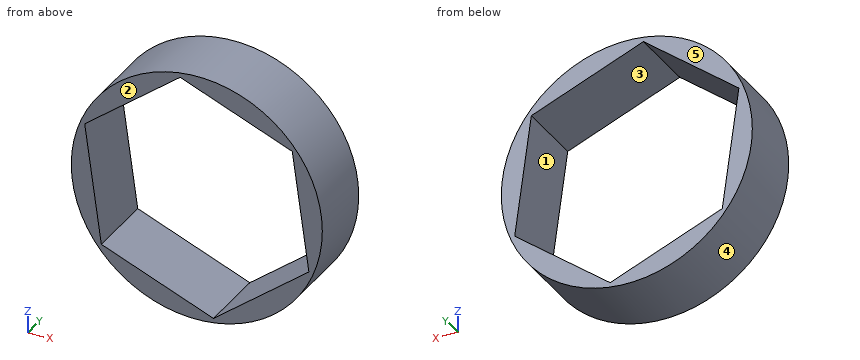
from build123d import *

# Parameters (mm, degrees)
F0_R     = 18
F1_DEPTH = 10


with BuildPart() as f1:
    # F0 (on Front) → F1 (new body)
    with BuildSketch(Plane.XZ):
        Circle(F0_R)
        Polygon((-16.075068, 6.526333), (-2.385564, 17.184584), (13.689504, 10.658251), (16.075068, -6.526333), (2.385564, -17.184584), (-13.689504, -10.658251), align=None, mode=Mode.SUBTRACT)
    extrude(amount=-F1_DEPTH)


solid = f1.part
Check sheet for the modelled part. Datum: model origin and axes. Units: mm. Face numbers are marked on the shaded views. A direction names the side the tool comes from. Give positions to 0.01 mm unless a question says otherwise; leave off trailing zeros. Write each loop counter-clockwise with the first axis right and the second up, starting at its lowest first coordinate (ties: lowest second). Pieces come first, ordered by that corner, then holes. Notation, with made-up numbers: (-10.75, 44) -> (-0.75, 44) arc R31 cw to (-0.75, 73) -> close; hole circle Ø5 at (-13, -36.5). An arc over 180 degrees is marked (long way). One line per item, written item: value. Start each with the question number.
Item 1: Section check B-B on z = 0. Record the cut outline in (x, y), then the cut area to 3 significant figures.
Item 2: Section check C-C on x = -5.5. Record the cut outline in (y, z).
Item 3: Draft check along Z on the marked faces 3, 4 and 5. Enter one of: +Z half, -Z half, draft (parallel to the pull), parting line (faces both ways), or undercut.
Item 4: Section check A-A on y = 7.25. Record the cut outline in (x, z), then the cut area to 3 significant figures.
Item 5: Gauge pin test, flat ends, axial feed: pin 1 (6 mm diameter, centred on x = 7.5, y = 6.5, fed in from -Z); pin 2 (4 mm diameter, centred on y = 4.5, z = -3, fed in from +X); pin 3 (5 mm diameter, centred on y = 3, z = -7, fed in from +X); pin 4 (4 mm diameter, centred on x = 12.5, z = 2.5, fed in from +Y). Record the tip position at first contact, or that the pin passes through.
Item 6: Tool access check on the marked faces 1 and 2. Record the directions out of +Z, -Z, +X, -X, +Y, -Y that give a thin tool (end or side, any length) a straight path to the whole face; none if there is none.
Item 7: Material ranges on probe 1 along X at (y, z) = (4, 5.5); probe 2 along X at (y, z) = (6, 9); probe 3 along Z at (x, y) = (-8, 2), recorded low to high. Write a range as from..to.
Results list:
1. outline: (-18, 0) -> (-15.17, 0) -> (-15.17, 10) -> (-18, 10) -> close; (15.17, 0) -> (18, 0) -> (18, 10) -> (15.17, 10) -> close
1. area: 56.6 mm²
2. outline: (0, -17.14) -> (10, -17.14) -> (10, -13.98) -> (0, -13.98) -> close; (0, 14.76) -> (10, 14.76) -> (10, 17.14) -> (0, 17.14) -> close
3. face 3: undercut
3. face 4: parting line
3. face 5: draft
4. outline: circle Ø36 at (0, 0); hole (-16.08, 6.53) -> (-13.69, -10.66) -> (2.39, -17.18) -> (16.08, -6.53) -> (13.69, 10.66) -> (-2.39, 17.18) -> close
4. area: 236 mm²
5. pin 1: z = -17.43
5. pin 2: x = 17.97
5. pin 3: x = 17.43
5. pin 4: through
6. face 1: +Y, -Y
6. face 2: +Z, -Z, +X, -X, -Y
7. probe 1: -17.14..-15.93, 14.41..17.14
7. probe 2: -15.59..-12.9, 13.92..15.59
7. probe 3: -16.12..-12.97, 12.81..16.12
